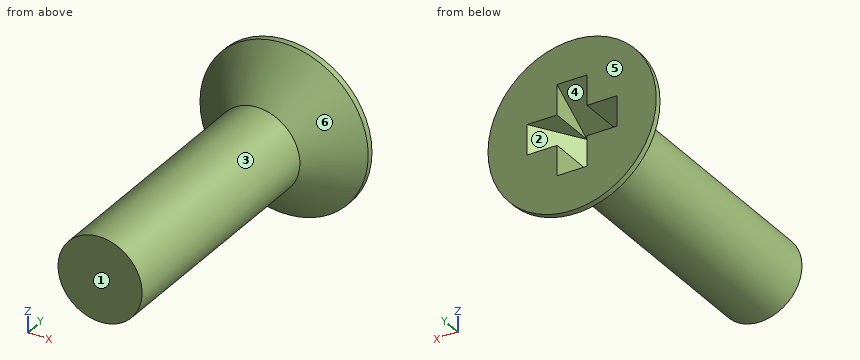
Autodesk Inventor part; units mm, degrees
ref_plane "YZ Plane" through (0, 0, 0) normal (1, 0, 0) x (0, 1, 0)
ref_plane "XZ Plane" through (0, 0, 0) normal (0, 1, 0) x (-1, 0, 0)
ref_plane "XY Plane" through (0, 0, 0) normal (0, 0, 1) x (1, 0, 0)
sketch "Эскиз1" plane through (0, 0, 0) normal (0, 0, 1) x (1, 0, 0)
  line L0 (-1.4, 0) -> (-1.4, -8.4)
  line L1 (-1.4, -8.4) -> (0, -8.4)
  line L2 (0, -8.4) -> (0, 1.6)
  line L3 (0, 1.6) -> (-2.8, 1.6)
  line L4 (-2.8, 1.6) -> (-2.8, 1.4)
  line L5 (-2.8, 1.4) -> (-1.4, 0)
  point P0 (0, 0)
  dimension "d0" = 2.8
  dimension "d2" = 45
  dimension "d3" = 1.6
  dimension "d4" = 10
  dimension "d5" = 5.6
revolve "Вращение1" add sketch "Эскиз1" angle 360 about axis through (0, -8.4, 0) along (0, 1, 0)
sketch "Эскиз2" plane through (0, 0, 0) normal (1, 0, 0) x (0, 1, 0)
  line L0 (1.6, -2.8) -> (1.6, 2.8)
  line L1 (1.6, 1.5) -> (1.6, 0)
  line L2 (0, 0) -> (1.6, 0)
  line L3 (1.6, 1.5) -> (0, 0.5)
  line L4 (0, -1.4) -> (0, 1.4)
  line L5 (0, 0) -> (0, 0.5)
  dimension "d7" = 1.5
  dimension "d13" = 0.5
extrude "Выдавливание1" cut sketch "Эскиз2" along normal mid plane 1
pattern_circular "Круговой массив1" count 4 over 360 about axis through (0, -10, 0) along (0, 1, 0) of "Выдавливание1"
thread "Резьба1"
properties part number "M3x10P"
Could you check a few things on this model? Use its own coordinates, in mm. Face numbers are marked on the shaded views. A direction names the side the tool comes from. Give positions to 0.01 mm unless a question says otherwise; leave off trailing zeros. Write each loop counter-clockwise with the first axis right and the second up, starting at its lowest first coordinate (ties: lowest second). Pieces come first, ordered by that corner, then holes. Notation, with made-up numbers: (9.5, 57) - (63.5, 57) arc R17 ccw to (63.5, 74) - close; hole circle Ø4 at (33.25, 24). An arc over 180 degrees is marked (long way). One line per item, written item: value. Start each with the question number.
Item 1: Imagine slicing it at D-D, the plane y = -2.75. List the corners of the cut face in (x, z) for me.
Item 2: I'm going to push flat-ended pins straight in: pin 1 (0.5 mm diameter, centred on x = 0, z = 0, fed in from +Y); pin 2 (1.1 mm diameter, centred on x = 1, y = 0.5, fed in from +Z); pin 3 (0.5 mm diameter, centred on x = -1, y = 0.5, fed in from -Z). Where does each tip first touch, or does it pass through?
Item 3: Which directions (+Z, -Z, +X, -X, +Y, -Y) give clear straight access to the entire face, cutting with the end or side of a thin tool? Please do the marked faces 1, 2 and 3.
Item 4: Imagine slicing it at C-C, the plane z = 0. List the corners of the cut face in (x, y) for me, and give its area (3 significant figures).
Item 5: If we mould it in two halves opening along X, with no side actions, what happens to the marked faces 4, 5 and 6? For each: +X half, -X half, draft (parallel to the pull), parting line (faces both ways), or undercut.
Item 6: Please list where these lines run through material, in increasing order: line 1 (Z direction, x = 0.7, y = 0.5); line 2 (X direction, y = 1, z = -0.55); line 3 (Z direction, x = 0, y = -6). Write a range as from..to.
Item 7: Imagine slicing it at B-B, the plane y = 0.75. List the corners of the cut face in (x, z) for me, and give its area (3 significant figures).
Item 8: Imagine slicing it at A-A, the plane x = 0. List the corners of the cut face in (y, z) for me.
Geometry says:
1. outline: circle Ø2.8 at (0, 0)
2. pin 1: y = 0
2. pin 2: z = 2.28
2. pin 3: z = -1.93
3. face 1: +Z, -Z, +X, -X, -Y
3. face 2: +Y
3. face 3: -Y
4. outline: (-2.8, 1.4) - (-1.4, 0) - (-1.4, -8.4) - (1.4, -8.4) - (1.4, 0) - (2.8, 1.4) - (2.8, 1.6) - (1.5, 1.6) - (0.5, 0) - (-0.5, 0) - (-1.5, 1.6) - (-2.8, 1.6) - close
4. area: 27.3 mm^2
5. face 4: undercut
5. face 5: draft
5. face 6: parting line
6. line 1: -1.77..-0.5, 0.5..1.77
6. line 2: -2.34..-0.5, 0.5..2.34
6. line 3: -1.4..1.4
7. outline: circle Ø4.3 at (0, 0); hole (-0.97, -0.5) - (-0.5, -0.5) - (-0.5, -0.97) - (0.5, -0.97) - (0.5, -0.5) - (0.97, -0.5) - (0.97, 0.5) - (0.5, 0.5) - (0.5, 0.97) - (-0.5, 0.97) - (-0.5, 0.5) - (-0.97, 0.5) - close
7. area: 11.6 mm^2
8. outline: (-8.4, -1.4) - (0, -1.4) - (1.4, -2.8) - (1.6, -2.8) - (1.6, -1.5) - (0, -0.5) - (0, 0.5) - (1.6, 1.5) - (1.6, 2.8) - (1.4, 2.8) - (0, 1.4) - (-8.4, 1.4) - close
